Could you check a few things on this model? Use its own coordinates, in mm. Round coordinates to 2 decimals unless told otherwise and drop trailing zeros. Loops run counter-clockwise (first coordinate to the right, second up) from the corner with the lowest first, then second, coordinate; pieces in that order, holes last. Notation, with made-up numbers: (4, 35) - (24, 35) arc R32 ccw to (24, 70) - close; hole circle Ø6 at (-1.75, 12.5). An arc over 180 degrees is marked (long way). Answer as CSV lines item,"result". Start each with the question number.
1) I'm going to push flat-ended pins straight in: pin 1 Ø4 at (x, z) = (23, -3) entering from -Y; pin 2 Ø1.5 at (x, y) = (69, 1) entering from +Z; pin 3 Ø1.2 at (x, y) = (24.5, -1.5) entering from -Z. Where does each tip first touch, or does it pass through?
2) Suppose I cut it at A-A, the plane x = 40. Write out the boundary of the cut face in (y, z).
3) Please list where these lines run through material, in increasing order: line 1 along Z through (x, y) = (49.5, -2); line 2 along Z through (x, y) = (62, -0.75).
```python
from build123d import *

# Parameters (mm, degrees)
F0_R          = 3
F1_DEPTH      = 96
F2_SIZE       = 0.5
F3_W          = 1
F3_H          = 1
F6_DEPTH      = 3.001
F6_DEPTH_BACK = 25
F8_DEPTH      = 0.75
F8_DEPTH_BACK = 0.75
F9_R          = 1.5


with BuildPart() as f1:
    # F0 (on Right) → F1 (new body)
    with BuildSketch(Plane.YZ):
        Circle(F0_R)
    extrude(amount=F1_DEPTH)

    # F2
    f2_edges = [f1.edges().sort_by_distance(p)[0] for p in [
        (0, -3, 0),
        (96, -3, 0),
    ]]
    chamfer(f2_edges, length=F2_SIZE)

    # F3 (on Front) → F4 (revolve, cut)
    with BuildSketch(Plane.XZ):
        with Locations((2, 3)):
            Rectangle(F3_W, F3_H)
        with Locations((94, 3)):
            Rectangle(F3_W, F3_H)
    revolve(axis=Axis((48.1495447457, 0, 0), (1, 0, 0)), mode=Mode.SUBTRACT)

    # F5 (on Front) → F6 (cut, two sides)
    with BuildSketch(Plane.XZ) as f6_sk:
        Polygon((26.5, 4), (22.5, 4), (22.5, 3), (23.5, 2), (25.5, 2), (26.5, 3), align=None)
        Polygon((26.5, -4), (26.5, -3), (25.5, -2), (23.5, -2), (22.5, -3), (22.5, -4), align=None)
    extrude(amount=-F6_DEPTH, mode=Mode.SUBTRACT)
    extrude(f6_sk.sketch, amount=F6_DEPTH_BACK, mode=Mode.SUBTRACT)

    # F7 (on Front) → F8 (join, two sides)
    with BuildSketch(Plane.XZ) as f8_sk:
        Polygon((22.5, 3), (22.5, 2), (26.5, 2), (26.5, 3), (25.5, 4), (23.5, 4), align=None)
        Polygon((22.5, -2), (22.5, -3), (23.5, -4), (25.5, -4), (26.5, -3), (26.5, -2), align=None)
    extrude(amount=F8_DEPTH)
    extrude(f8_sk.sketch, amount=-F8_DEPTH_BACK)

    # F9
    f9_edges = [f1.edges().sort_by_distance(p)[0] for p in [
        (23.5, 0, -4),
        (25.5, 0, -4),
        (23.5, 0, 4),
        (25.5, 0, 4),
    ]]
    fillet(f9_edges, radius=F9_R)


solid = f1.part
```
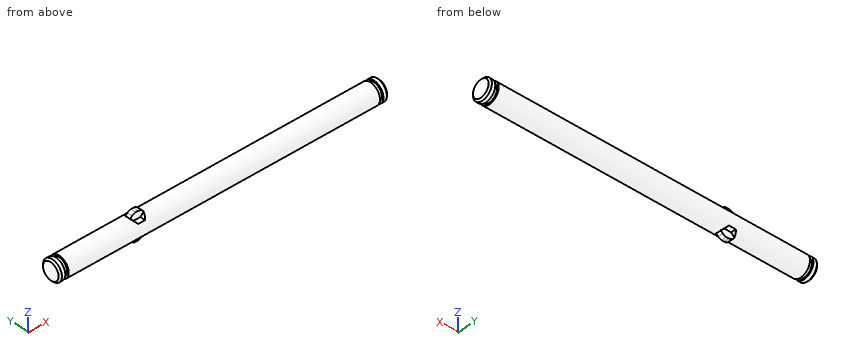
Filled sheet:
1,pin 1,"y = -2.83"
1,pin 2,"z = 2.99"
1,pin 3,"z = -2"
2,outline,"circle Ø6 at (0, 0)"
3,line 1,"-2.24 to 2.24"
3,line 2,"-2.9 to 2.9"
